from build123d import *

# Parameters (mm, degrees)
SKETCH1_W                                            = 340
SKETCH1_H                                            = 150
BOSS_EXTRUDE1_DEPTH                                  = 20
LASERCAVITYMOUNTINGHOLE_CBORE_FOR_1_4_SO_D           = 6.7564
LASERCAVITYMOUNTINGHOLE_CBORE_FOR_1_4_SO_CBORE_D     = 11.1125
LASERCAVITYMOUNTINGHOLE_CBORE_FOR_1_4_SO_CBORE_DEPTH = 6.35
SKETCH5_W                                            = 57
SKETCH5_H                                            = 57
TEC_GROOVE_DEPTH                                     = 1
SKETCH6_W                                            = 340
SKETCH6_H                                            = 8
WALL1_DEPTH                                          = 8
SKETCH7_W                                            = 142
SKETCH7_H                                            = 8
WALL2_DEPTH                                          = 8
SKETCH9_W                                            = 332
SKETCH9_H                                            = 8
WALL3_DEPTH                                          = 8
SKETCH10_W                                           = 134
SKETCH10_H                                           = 8
WALL4_DEPTH                                          = 8
F_2_56_TAPPED_HOLE1_D                                = 1.778
F_2_56_TAPPED_HOLE1_DEPTH                            = 15
F_2_56_TAPPED_HOLE1_TIP                              = 0.53416509
F_2_56_TAPPED_HOLE2_D                                = 1.778
F_2_56_TAPPED_HOLE2_DEPTH                            = 15
F_2_56_TAPPED_HOLE2_TIP                              = 0.53416509
F_2_56_TAPPED_HOLE3_D                                = 1.778
F_2_56_TAPPED_HOLE3_DEPTH                            = 15
F_2_56_TAPPED_HOLE3_TIP                              = 0.53416509
ELECTRONICBOARDMOUNTING_D                            = 2.2606
ELECTRONICBOARDMOUNTING_DEPTH                        = 20
ELECTRONICBOARDMOUNTING_TIP                          = 0.679152758
F_2_56_TAPPED_HOLE4_D                                = 1.778
F_2_56_TAPPED_HOLE4_DEPTH                            = 15
F_2_56_TAPPED_HOLE4_TIP                              = 0.53416509
OPTICALTABLEMOUNTINGHOLES_CBORE_FOR_1_4_D            = 6.7564
OPTICALTABLEMOUNTINGHOLES_CBORE_FOR_1_4_DEPTH        = 20
OPTICALTABLEMOUNTINGHOLES_CBORE_FOR_1_4_CBORE_D      = 14.2875
OPTICALTABLEMOUNTINGHOLES_CBORE_FOR_1_4_CBORE_DEPTH  = 4.191
OPTICALTABLEMOUNTINGHOLES_CBORE_FOR_1_4_TIP          = 2.029827343


with BuildPart() as part:
    # Sketch1 → Boss-Extrude1 (new body)
    with BuildSketch(Plane(origin=(0, 0, 0), x_dir=(1, 0, 0), z_dir=(0, 1, 0))):
        with Locations((170, 75)):
            Rectangle(SKETCH1_W, SKETCH1_H)
    extrude(amount=BOSS_EXTRUDE1_DEPTH)

    # LaserCavityMountingHole_CBORE for 1/4 Socket Head Cap Screw1 (through all)
    with Locations(Plane(origin=(0, 0, 0), x_dir=(-1, 0, 0), z_dir=(0, -1, 0))):
        with Locations((-100, 40), (-190, 40), (-280, 40), (-280, 110), (-190, 110), (-100, 110)):
            CounterBoreHole(LASERCAVITYMOUNTINGHOLE_CBORE_FOR_1_4_SO_D / 2, LASERCAVITYMOUNTINGHOLE_CBORE_FOR_1_4_SO_CBORE_D / 2, LASERCAVITYMOUNTINGHOLE_CBORE_FOR_1_4_SO_CBORE_DEPTH)

    # Sketch5 → TEC_groove (cut)
    with BuildSketch(Plane(origin=(0, 20, 0), x_dir=(1, 0, 0), z_dir=(0, 1, 0))):
        with Locations((140, 75)):
            Rectangle(SKETCH5_W, SKETCH5_H)
        with Locations((240, 75)):
            Rectangle(SKETCH5_W, SKETCH5_H)
    extrude(amount=-TEC_GROOVE_DEPTH, mode=Mode.SUBTRACT)

    # Sketch6 → Wall1 (cut)
    with BuildSketch(Plane.XY):
        with Locations((170, 16)):
            Rectangle(SKETCH6_W, SKETCH6_H)
    extrude(amount=-WALL1_DEPTH, mode=Mode.SUBTRACT)

    # Sketch7 → Wall2 (cut)
    with BuildSketch(Plane(origin=(340, 0, 0), x_dir=(0, 0, -1), z_dir=(1, 0, 0))):
        with Locations((79, 16)):
            Rectangle(SKETCH7_W, SKETCH7_H)
    extrude(amount=-WALL2_DEPTH, mode=Mode.SUBTRACT)

    # Sketch9 → Wall3 (cut)
    with BuildSketch(Plane(origin=(0, 0, -150), x_dir=(-1, 0, 0), z_dir=(0, 0, -1))):
        with Locations((-166, 16)):
            Rectangle(SKETCH9_W, SKETCH9_H)
    extrude(amount=-WALL3_DEPTH, mode=Mode.SUBTRACT)

    # Sketch10 → Wall4 (cut)
    with BuildSketch(Plane.ZY):
        with Locations((-75, 16)):
            Rectangle(SKETCH10_W, SKETCH10_H)
    extrude(amount=-WALL4_DEPTH, mode=Mode.SUBTRACT)

    # #2-56 Tapped Hole1
    with Locations(Plane.XY.offset(-8)):
        with Locations((18, 16), (322, 16), (170, 16)):
            Hole(F_2_56_TAPPED_HOLE1_D / 2, depth=F_2_56_TAPPED_HOLE1_DEPTH)
            with Locations((0, 0, -(F_2_56_TAPPED_HOLE1_DEPTH + F_2_56_TAPPED_HOLE1_TIP / 2))):  # 118° drill point
                Cone(0, F_2_56_TAPPED_HOLE1_D / 2, F_2_56_TAPPED_HOLE1_TIP, mode=Mode.SUBTRACT)

    # #2-56 Tapped Hole2
    with Locations(Plane(origin=(8, 16, -132), x_dir=(0, 0, -1), z_dir=(-1, 0, 0))):
        with Locations((0, 0), (-114, 0), (-57, 0)):
            Hole(F_2_56_TAPPED_HOLE2_D / 2, depth=F_2_56_TAPPED_HOLE2_DEPTH)
            with Locations((0, 0, -(F_2_56_TAPPED_HOLE2_DEPTH + F_2_56_TAPPED_HOLE2_TIP / 2))):  # 118° drill point
                Cone(0, F_2_56_TAPPED_HOLE2_D / 2, F_2_56_TAPPED_HOLE2_TIP, mode=Mode.SUBTRACT)

    # #2-56 Tapped Hole3
    with Locations(Plane(origin=(0, 0, -142), x_dir=(-1, 0, 0), z_dir=(0, 0, -1))):
        with Locations((-322, 16), (-18, 16), (-170, 16)):
            Hole(F_2_56_TAPPED_HOLE3_D / 2, depth=F_2_56_TAPPED_HOLE3_DEPTH)
            with Locations((0, 0, -(F_2_56_TAPPED_HOLE3_DEPTH + F_2_56_TAPPED_HOLE3_TIP / 2))):  # 118° drill point
                Cone(0, F_2_56_TAPPED_HOLE3_D / 2, F_2_56_TAPPED_HOLE3_TIP, mode=Mode.SUBTRACT)

    # ElectronicBoardMounting
    with Locations(Plane(origin=(0, 20, 0), x_dir=(1, 0, 0), z_dir=(0, 1, 0))):
        with Locations((187, 127), (277, 127), (277, 77), (187, 77)):
            Hole(ELECTRONICBOARDMOUNTING_D / 2, depth=ELECTRONICBOARDMOUNTING_DEPTH)
            with Locations((0, 0, -(ELECTRONICBOARDMOUNTING_DEPTH + ELECTRONICBOARDMOUNTING_TIP / 2))):  # 118° drill point
                Cone(0, ELECTRONICBOARDMOUNTING_D / 2, ELECTRONICBOARDMOUNTING_TIP, mode=Mode.SUBTRACT)

    # #2-56 Tapped Hole4
    with Locations(Plane(origin=(332, 0, 0), x_dir=(0, 0, -1), z_dir=(1, 0, 0))):
        with Locations((18, 16), (132, 16), (75, 16)):
            Hole(F_2_56_TAPPED_HOLE4_D / 2, depth=F_2_56_TAPPED_HOLE4_DEPTH)
            with Locations((0, 0, -(F_2_56_TAPPED_HOLE4_DEPTH + F_2_56_TAPPED_HOLE4_TIP / 2))):  # 118° drill point
                Cone(0, F_2_56_TAPPED_HOLE4_D / 2, F_2_56_TAPPED_HOLE4_TIP, mode=Mode.SUBTRACT)

    # OpticalTableMountingHoles_CBORE for 1/4 Binding Head Machine Screw1
    with Locations(Plane(origin=(0, 20, 0), x_dir=(1, 0, 0), z_dir=(0, 1, 0))):
        with Locations((63, 109.6), (317, 109.6), (317, 33.4), (63, 33.4)):
            CounterBoreHole(OPTICALTABLEMOUNTINGHOLES_CBORE_FOR_1_4_D / 2, OPTICALTABLEMOUNTINGHOLES_CBORE_FOR_1_4_CBORE_D / 2, OPTICALTABLEMOUNTINGHOLES_CBORE_FOR_1_4_CBORE_DEPTH, depth=OPTICALTABLEMOUNTINGHOLES_CBORE_FOR_1_4_DEPTH)
            with Locations((0, 0, -(OPTICALTABLEMOUNTINGHOLES_CBORE_FOR_1_4_DEPTH + OPTICALTABLEMOUNTINGHOLES_CBORE_FOR_1_4_TIP / 2))):  # 118° drill point
                Cone(0, OPTICALTABLEMOUNTINGHOLES_CBORE_FOR_1_4_D / 2, OPTICALTABLEMOUNTINGHOLES_CBORE_FOR_1_4_TIP, mode=Mode.SUBTRACT)


solid = part.part
Build history of the part. All positions in model axes, mm. A direction names the side the tool comes from. Give positions to 0.01 mm unless a question says otherwise; leave off trailing zeros. Loops run counter-clockwise (first coordinate to the right, second up) from the corner with the lowest first, then second, coordinate; pieces in that order, holes last. Notation, with made-up numbers: (-7, 83.5) - (0, 83.5) arc R13 ccw to (0, 94.5) - close; hole circle Ø1 at (74.5, 73). An arc over 180 degrees is marked (long way). Write item = value, one per line. Start each with the question number.
1) Tool access for faces 4 (the flat face through (100, 6.35, -106)), 5 (the flat face through (8, 15, -76)), 6 (the cylindrical face through (61.184, 7.794, -112.449)), 7 (the flat face through (340, 6, -74)), 8 (the flat face through (140, 19, -75)): list every direction of +Z, -Z, +X, -X, +Y, -Y with a clear straight run to the whole face (end or side of a thin tool).
2) Probe probe 1 along Z at (x, y) = (100, 9.25); probe 2 along X at (y, z) = (16, -129.5); probe 3 along Z at (x, y) = (63, 5). List the from-to ranges inside material, lowest first. Write a range as from..to.
3) Drop flat-ended pins along their axis: pin 1 Ø3 at (x, y) = (215, 15.5) entering from +Z; pin 2 Ø9 at (x, z) = (101, -42) entering from -Y; pin 3 Ø10 at (x, z) = (100, -40) entering from -Y; pin 4 Ø1.1 at (y, z) = (16, -132) entering from +X. Give the stop position or say it passes through.
4) Pull direction X, two halves, no side cores. Call faces 1 (the flat face through (0, 6, -74)), 2 (the flat face through (64, 15.809, -30)), 3 (the flat face through (168, 16, -8)): +X half, -X half, draft (parallel to the pull), parting line (faces both ways), or undercut.
5) Band-saw the part on A-A on x = 100. Give the cut face in (y, z).
6) Band-saw the part on C-C on x = 246.5. Give the cut face in (y, z), plus the area to 4 significant figures.
7) Band-saw the part on D-D on x = 176. Give the cut face in (y, z).
8) Band-saw the part on B-B on z = -51.5. Give the cut face in (x, y), plus the area to 3 significant figures.
Final values:
q1.face_4 = -Y
q1.face_5 = +Z, -Z, -X, +Y
q1.face_6 = +Y, -Y
q1.face_7 = +Z, -Z, +X, +Y, -Y
q1.face_8 = +Y
q2.probe_1 = -150..-113.38, -106.62..-43.38, -36.62..0
q2.probe_2 = 8..17.11, 18.89..169.11, 170.89..321.11, 322.89..332
q2.probe_3 = -150..-112.98, -106.22..-36.78, -30.02..0
q3.pin_1 = -8
q3.pin_2 = 0
q3.pin_3 = 6.35
q3.pin_4 = 316.8
q4.face_1 = -X half
q4.face_2 = undercut
q4.face_3 = draft
q5.outline = (0, -150) - (12, -150) - (12, -142) - (20, -142) - (20, -113.38) - (6.35, -113.38) - (6.35, -115.56) - (0, -115.56) - close; (0, -104.44) - (6.35, -104.44) - (6.35, -106.62) - (20, -106.62) - (20, -43.38) - (6.35, -43.38) - (6.35, -45.56) - (0, -45.56) - close; (0, -34.44) - (6.35, -34.44) - (6.35, -36.62) - (20, -36.62) - (20, -8) - (12, -8) - (12, 0) - (0, 0) - close
q6.outline = (0, -150) - (12, -150) - (12, -142) - (20, -142) - (20, -103.5) - (19, -103.5) - (19, -46.5) - (20, -46.5) - (20, -8) - (12, -8) - (12, 0) - (0, 0) - close
q6.area = 2,815 mm²
q7.outline = (0, -150) - (12, -150) - (12, -142) - (20, -142) - (20, -8) - (12, -8) - (12, 0) - (0, 0) - close
q8.outline = (0, 0) - (340, 0) - (340, 12) - (332, 12) - (332, 20) - (268.5, 20) - (268.5, 19) - (211.5, 19) - (211.5, 20) - (168.5, 20) - (168.5, 19) - (111.5, 19) - (111.5, 20) - (8, 20) - (8, 12) - (0, 12) - close
q8.area = 6,560 mm²
